Input: part model. Units: mm. Frame: model coordinates. Face numbers are marked on the shaded views. A direction names the side the tool comes from. Give positions to 0.01 mm unless a question says otherwise; leave off trailing zeros. Write each loop counter-clockwise with the first axis right and the second up, starting at its lowest first coordinate (ties: lowest second). Pieces come first, ordered by that corner, then holes. Notation, with made-up numbers: (24.25, 38.5) -> (55.25, 38.5) arc R9 ccw to (55.25, 48.5) -> close; hole circle Ø4 at (42.25, -37.75). An arc over 180 degrees is marked (long way). Return JSON: item names as keys, results as strings. Group by question number.
Item 1: Section C-C, the plane x = 15. Return loops of the section in (y, z), then the cut area to 3 significant figures.
Item 2: Pin query (flat end, axial travel): P1, Ø8, axis at y = -13, z = 9.5, coming from the +X side; P2, Ø9, axis at x = -2, y = -2.5, coming from the -Z side; P3, Ø6, axis at x = -15, z = 22, coming from the -Y side; P4, Ø1, axis at x = -22.5, y = 10, coming from the -Z side. Return the tip coordinate at first contact, or that it passes through.
Item 3: Line query: line 1 (Y direction, x = 0, z = 35); line 2 (Z direction, x = 9.5, y = -0.5); line 3 (Y direction, x = 0, z = 17.25). Output: solid intervals per line, ascending. Write a range as [from, to].
Item 4: Set-up query: the marked faces 4 and 5. Return all of +Z, -Z, +X, -X, +Y, -Y with unobstructed straight access to the full face (end or side cutting, diameter ignored); none if empty.
Item 5: Section A-A, the plane z = 26. Return loops of the section in (x, y).
Item 6: Mould query, pull axis Y, two halves, no side actions, for the marked faces 1, 2 and 3. Classes: released by +Y, released by -Y, zero draft, split by the parting line, or undercut.
Item 7: Section B-B, the plane y = 0. Return loops of the section in (x, z).
Item 8: Section D-D, the plane x = 0. Return loops of the section in (y, z).
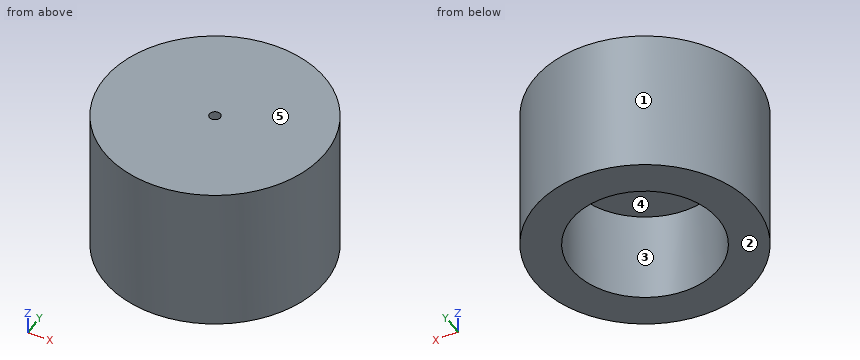
from build123d import *

# Parameters (mm, degrees)
SKETCH1_R           = 30
BOSS_EXTRUDE1_DEPTH = 40
SKETCH2_R           = 20
CUT_EXTRUDE1_DEPTH  = 25
CUT_EXTRUDE2_DEPTH  = 5
SKETCH5_R           = 1.5
CUT_EXTRUDE3_DEPTH  = 40


with BuildPart() as part:
    # Sketch1 → Boss-Extrude1 (new body)
    with BuildSketch(Plane.XY):
        Circle(SKETCH1_R)
    extrude(amount=BOSS_EXTRUDE1_DEPTH)

    # Sketch2 → Cut-Extrude1 (cut)
    with BuildSketch(Plane(origin=(0, 0, 0), x_dir=(-1, 0, 0), z_dir=(0, 0, -1))):
        Circle(SKETCH2_R)
    extrude(amount=-CUT_EXTRUDE1_DEPTH, mode=Mode.SUBTRACT)

    # Sketch3 → Cut-Extrude2 (cut)
    with BuildSketch(Plane(origin=(0, 0, 25), x_dir=(-1, 0, 0), z_dir=(0, 0, -1))):
        Polygon((4.082774554, -4.396697846), (5.849039304, 1.337437558), (1.76626475, 5.734135404), (-4.082774554, 4.396697846), (-5.849039304, -1.337437558), (-1.76626475, -5.734135404), align=None)
    extrude(amount=-CUT_EXTRUDE2_DEPTH, mode=Mode.SUBTRACT)

    # Sketch5 → Cut-Extrude3 (cut)
    with BuildSketch(Plane.XY.offset(40)):
        Circle(SKETCH5_R)
    extrude(amount=-CUT_EXTRUDE3_DEPTH, mode=Mode.SUBTRACT)


solid = part.part
Answer below:
{
 "1": {"outline": "(-25.98, 0) -> (-13.23, 0) -> (-13.23, 25) -> (13.23, 25) -> (13.23, 0) -> (25.98, 0) -> (25.98, 40) -> (-25.98, 40) -> close", "area": "1,420 mm2"},
 "2": {"P1": "stops at x = 28.62", "P2": "stops at z = 25", "P3": "stops at y = -27.5", "P4": "stops at z = 0"},
 "3": {"line 1": "y = [-30, -1.5], [1.5, 30]", "line 2": "z = [25, 40]", "line 3": "y = [-30, -20], [20, 30]"},
 "4": {"face 4": "-Z", "face 5": "+Z, +X, -X, +Y, -Y"},
 "5": {"outline": "circle Ø60 at (0, 0); hole (-5.85, 1.34) -> (-4.08, -4.4) -> (1.77, -5.73) -> (5.85, -1.34) -> (4.08, 4.4) -> (-1.77, 5.73) -> close"},
 "6": {"face 1": "split by the parting line", "face 2": "zero draft", "face 3": "undercut"},
 "7": {"outline": "(-30, 0) -> (-20, 0) -> (-20, 25) -> (-5.44, 25) -> (-5.44, 30) -> (-1.5, 30) -> (-1.5, 40) -> (-30, 40) -> close; (1.5, 30) -> (5.44, 30) -> (5.44, 25) -> (20, 25) -> (20, 0) -> (30, 0) -> (30, 40) -> (1.5, 40) -> close"},
 "8": {"outline": "(-30, 0) -> (-20, 0) -> (-20, 25) -> (-5.33, 25) -> (-5.33, 30) -> (-1.5, 30) -> (-1.5, 40) -> (-30, 40) -> close; (1.5, 30) -> (5.33, 30) -> (5.33, 25) -> (20, 25) -> (20, 0) -> (30, 0) -> (30, 40) -> (1.5, 40) -> close"}
}
